Could you check a few things on this drawing? It's one solid part, dimensions in mm from its lowest x, y, z. Give positions to 0.01 mm unless a question says otherwise; leave off trailing zeros. Order: outer loops, then holes, each group sorted by start corner. A loop starts at its lowest first (then second) coordinate and runs counter-clockwise, first axis right, second up. Notation, with made-up numbers: (-5, 8) -> (39, 8) arc R22 ccw to (39, 25) -> close; hole circle Ø9 at (-25.75, 79). An arc over 180 degrees is marked (long way). Answer as a JSON object with one key per item and string values.
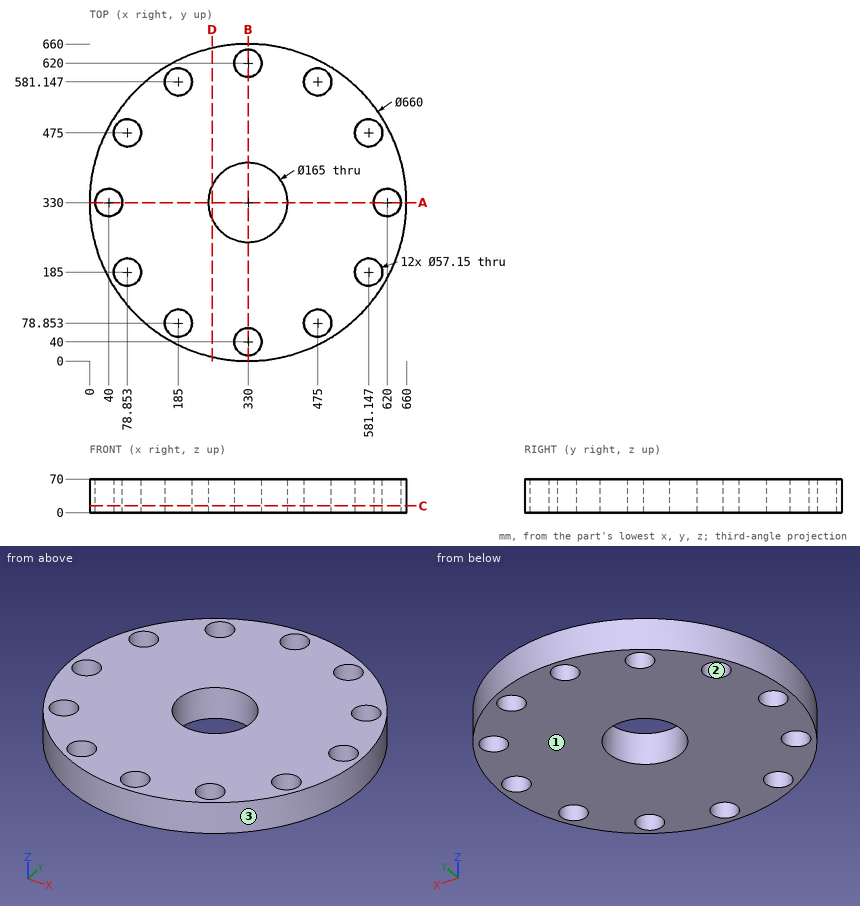
1. Will these pins go through, and if not, where does the flat tip stop? pin 1 Ø1.5 at (x, z) = (126, 35.5) entering from +Y; pin 2 Ø5 at (x, z) = (101.5, 26.5) entering from +Y (1 decimal); pin 3 Ø8 at (x, z) = (216, 8.5) entering from -Y.
Worked answers:
{"pin 1": "y = 589.98", "pin 2": "y = 570.5", "pin 3": "y = 18.87"}
2. If we mould it in two halves opening along X, with no side actions, what happens to the marked faces 1, 2 and 3? For each: +X half, -X half, draft (parallel to the pull), parting line (faces both ways), or undercut.
Worked answers:
{"face 1": "draft", "face 2": "undercut", "face 3": "parting line"}
3. If we section it at D-D on x = 255.5: Please give me the cut outline in (y, z), then the cut area to 3 significant figures.
Worked answers:
{"outline": "(8.52, 0) -> (294.56, 0) -> (294.56, 70) -> (8.52, 70) -> close; (365.44, 0) -> (651.48, 0) -> (651.48, 70) -> (365.44, 70) -> close", "area": "40,000 mm²"}
4. If we section it at A-A on y = 330: Please give me the cut outline in (x, z) (1 decimal), then the cut area to 4 significant figures.
Worked answers:
{"outline": "(0, 0) -> (11.4, 0) -> (11.4, 70) -> (0, 70) -> close; (68.6, 0) -> (247.5, 0) -> (247.5, 70) -> (68.6, 70) -> close; (412.5, 0) -> (591.4, 0) -> (591.4, 70) -> (412.5, 70) -> close; (648.6, 0) -> (660, 0) -> (660, 70) -> (648.6, 70) -> close", "area": "26,650 mm²"}
5. If we section it at C-C on z = 14: Count the separate pieces of the cut face and the enclosed holes in it, then the cut area to 3 significant figures.
Worked answers:
{"separate pieces": "1", "enclosed holes": "13", "area": "290,000 mm²"}
6. Please list where these lines run through material, in increasing order: L1, parallel to Y at x = 330, z = 36 (1 decimal); L2, parallel to Y at x = 91.5, z = 50 (1 decimal); L3, parallel to Y at x = 476, z = 4 (1 decimal).
Worked answers:
{"L1": "0 to 11.4, 68.6 to 247.5, 412.5 to 591.4, 648.6 to 660", "L2": "101.9 to 159.4, 210.6 to 449.4, 500.6 to 558.1", "L3": "34.1 to 50.3, 107.4 to 552.6, 609.7 to 625.9"}
